from build123d import *

# Parameters (mm, degrees)
SKETCH1_R               = 15.875
SKETCH1_R_2             = 3.25
BOSS_EXTRUDE1_DEPTH     = 12.7
BOSS_EXTRUDE2_START     = -12.7
SKETCH1_3_W             = 38.1
SKETCH1_3_H             = 31.75
SKETCH1_3_R             = 3.25
BOSS_EXTRUDE2_DEPTH     = 12.7
CUT_EXTRUDE1_REACH      = 41.144
CUT_EXTRUDE1_END_RADIUS = 3.25
BOSS_EXTRUDE3_DEPTH     = 31.75
FILLET1_R               = 15.875
SKETCH8_R               = 6.35
CUT_EXTRUDE3_DEPTH      = 76.282979766
SKETCH8_3_R             = 9.5
SKETCH8_3_R_2           = 6.35
CUT_EXTRUDE4_DEPTH      = 6
SKETCH9_R               = 6.35
SKETCH9_R_2             = 5.5
BOSS_EXTRUDE4_DEPTH     = 13.05
SKETCH10_R              = 1.95
CUT_EXTRUDE5_DEPTH      = 10.16
CUT_EXTRUDE6_REACH      = 102.653
CUT_EXTRUDE6_END_RADIUS = 5.5


with BuildPart() as part:
    # Sketch1 → Boss-Extrude1 (new body)
    with BuildSketch(Plane.XY):
        Circle(SKETCH1_R)
        Circle(SKETCH1_R_2, mode=Mode.SUBTRACT)
    extrude(amount=BOSS_EXTRUDE1_DEPTH)

    # Sketch1<3> → Boss-Extrude2 (add)
    with BuildSketch(Plane.XY.offset(BOSS_EXTRUDE2_START)):
        Rectangle(SKETCH1_3_W, SKETCH1_3_H)
        Circle(SKETCH1_3_R, mode=Mode.SUBTRACT)
    extrude(amount=BOSS_EXTRUDE2_DEPTH)

    # Cut-Extrude1: up to this cylinder (the profile starts outside it)
    cut_extrude1_end = Plane(origin=(0, 0, 6.35), z_dir=(0, 0, -1)) * Cylinder(CUT_EXTRUDE1_END_RADIUS, 89.788, mode=Mode.PRIVATE)
    # Sketch4 → Cut-Extrude1 (cut, up to the surface)
    with BuildSketch(Plane(origin=(0, 15.875, 0), x_dir=(1, 0, 0), z_dir=(0, 1, 0)), mode=Mode.PRIVATE) as cut_extrude1_sk1:
        with BuildLine():
            ThreePointArc((1.95, -6.35), (1.378858223, -4.971141777), (0, -4.4))
            Line((0, -4.4), (0, -8.3))
            ThreePointArc((0, -8.3), (1.378858223, -7.728858223), (1.95, -6.35))
        make_face()
    cut_extrude1_tool1 = extrude(cut_extrude1_sk1.sketch, amount=-CUT_EXTRUDE1_REACH, mode=Mode.PRIVATE) - cut_extrude1_end
    add(cut_extrude1_tool1.solids().sort_by_distance((0.827606, 15.875, 6.35))[0], mode=Mode.SUBTRACT)
    # Sketch4 → Cut-Extrude1 (cut, up to the surface)
    with BuildSketch(Plane(origin=(0, 15.875, 0), x_dir=(1, 0, 0), z_dir=(0, 1, 0)), mode=Mode.PRIVATE) as cut_extrude1_sk2:
        with BuildLine():
            Line((0, -8.3), (0, -4.4))
            ThreePointArc((0, -4.4), (-1.95, -6.35), (0, -8.3))
        make_face()
    cut_extrude1_tool2 = extrude(cut_extrude1_sk2.sketch, amount=-CUT_EXTRUDE1_REACH, mode=Mode.PRIVATE) - cut_extrude1_end
    add(cut_extrude1_tool2.solids().sort_by_distance((-0.827606, 15.875, 6.35))[0], mode=Mode.SUBTRACT)
    # Sketch4 → Cut-Extrude1 (cut, up to the surface)
    with BuildSketch(Plane(origin=(0, 15.875, 0), x_dir=(1, 0, 0), z_dir=(0, 1, 0)), mode=Mode.PRIVATE) as cut_extrude1_sk3:
        with BuildLine():
            ThreePointArc((1.95, -6.35), (1.378858223, -4.971141777), (0, -4.4))
            Line((0, -4.4), (0, -8.3))
            ThreePointArc((0, -8.3), (1.378858223, -7.728858223), (1.95, -6.35))
        make_face()
    cut_extrude1_tool3 = extrude(cut_extrude1_sk3.sketch, amount=-CUT_EXTRUDE1_REACH, mode=Mode.PRIVATE) - cut_extrude1_end
    add(cut_extrude1_tool3.solids().sort_by_distance((0.827606, 15.875, 6.35))[0], mode=Mode.SUBTRACT)
    # Sketch4 → Cut-Extrude1 (cut, up to the surface)
    with BuildSketch(Plane(origin=(0, 15.875, 0), x_dir=(1, 0, 0), z_dir=(0, 1, 0)), mode=Mode.PRIVATE) as cut_extrude1_sk4:
        with BuildLine():
            Line((0, -8.3), (0, -4.4))
            ThreePointArc((0, -4.4), (-1.95, -6.35), (0, -8.3))
        make_face()
    cut_extrude1_tool4 = extrude(cut_extrude1_sk4.sketch, amount=-CUT_EXTRUDE1_REACH, mode=Mode.PRIVATE) - cut_extrude1_end
    add(cut_extrude1_tool4.solids().sort_by_distance((-0.827606, 15.875, 6.35))[0], mode=Mode.SUBTRACT)

    # Sketch7 → Boss-Extrude3 (add)
    with BuildSketch(Plane(origin=(0, 15.875, 0), x_dir=(1, 0, 0), z_dir=(0, 1, 0))):
        with BuildLine():
            ThreePointArc((-19.05, 12.7), (-23.740191201, 19.121901724), (-25.4, 26.899031657))
            Line((-25.4, 26.899031657), (-25.4, 58.649031657))
            Line((-25.4, 58.649031657), (-44.45, 58.649031657))
            Line((-44.45, 58.649031657), (-44.45, 31.75))
            ThreePointArc((-44.45, 31.75), (-37.318649317, 11.420080546), (-19.05, 0))
            Line((-19.05, 0), (-19.05, 12.7))
        make_face()
    extrude(amount=-BOSS_EXTRUDE3_DEPTH)

    # Fillet1
    fillet1_edges = [part.edges().sort_by_distance(p)[0] for p in [
        (-34.925, -15.875, -58.649031657),
        (-34.925, 15.875, -58.649031657),
    ]]
    fillet(fillet1_edges, radius=FILLET1_R - 0.0001)  # a hair under: the kernel refuses the full size

    # Sketch8 → Cut-Extrude3 (cut, through all)
    with BuildSketch(Plane(origin=(-25.4, 0, 0), x_dir=(0, 0, -1), z_dir=(1, 0, 0))):
        with Locations((42.774031657, 0)):
            Circle(SKETCH8_R)
    extrude(amount=-CUT_EXTRUDE3_DEPTH, mode=Mode.SUBTRACT)

    # Sketch8<3> → Cut-Extrude4 (cut)
    with BuildSketch(Plane(origin=(-25.4, 0, 0), x_dir=(0, 0, -1), z_dir=(1, 0, 0))):
        with Locations((42.774031657, 0)):
            Circle(SKETCH8_3_R)
        with Locations((42.774031657, 0)):
            Circle(SKETCH8_3_R_2, mode=Mode.SUBTRACT)
    extrude(amount=-CUT_EXTRUDE4_DEPTH, mode=Mode.SUBTRACT)

    # Mirror1: part across plane


with BuildPart() as part_1:
    add(part.part)
    add(part.part.mirror(Plane(origin=(0, 0, 0), x_dir=(0, 0, 1), z_dir=(1, 0, 0))))

    # Sketch9 → Boss-Extrude4 (add)
    with BuildSketch(Plane(origin=(44.45, 0, 0), x_dir=(0, 0, -1), z_dir=(1, 0, 0))):
        with Locations((42.774031657, 0)):
            Circle(SKETCH9_R)
        with Locations((42.774031657, 0)):
            Circle(SKETCH9_R_2, mode=Mode.SUBTRACT)
    extrude(amount=-BOSS_EXTRUDE4_DEPTH)

    # Sketch10 → Cut-Extrude5 (cut)
    with BuildSketch(Plane.ZY.offset(44.45)):
        with Locations((-42.774031657, 12.7)):
            Circle(SKETCH10_R)
        with Locations((-42.774031657, -12.7)):
            Circle(SKETCH10_R)
    extrude(amount=-CUT_EXTRUDE5_DEPTH, mode=Mode.SUBTRACT)

    # Cut-Extrude6: up to this cylinder (the profile starts outside it)
    cut_extrude6_end = Plane(origin=(35.381138, 0, -42.774031657), z_dir=(1, 0, 0)) * Cylinder(CUT_EXTRUDE6_END_RADIUS, 217.306, mode=Mode.PRIVATE)
    # Sketch11 → Cut-Extrude6 (cut, up to the surface)
    with BuildSketch(Plane.XY.offset(-76.2), mode=Mode.PRIVATE) as cut_extrude6_sk1:
        with BuildLine():
            ThreePointArc((33.431138122, 0), (35.381138122, -1.95), (37.331138122, 0))
            Line((37.331138122, 0), (33.431138122, 0))
        make_face()
    cut_extrude6_tool1 = extrude(cut_extrude6_sk1.sketch, amount=CUT_EXTRUDE6_REACH, mode=Mode.PRIVATE) - cut_extrude6_end
    add(cut_extrude6_tool1.solids().sort_by_distance((35.381138, -0.827606, -76.2))[0], mode=Mode.SUBTRACT)
    # Sketch11 → Cut-Extrude6 (cut, up to the surface)
    with BuildSketch(Plane.XY.offset(-76.2), mode=Mode.PRIVATE) as cut_extrude6_sk2:
        with BuildLine():
            Line((33.431138122, 0), (37.331138122, 0))
            ThreePointArc((37.331138122, 0), (35.381138122, 1.95), (33.431138122, 0))
        make_face()
    cut_extrude6_tool2 = extrude(cut_extrude6_sk2.sketch, amount=CUT_EXTRUDE6_REACH, mode=Mode.PRIVATE) - cut_extrude6_end
    add(cut_extrude6_tool2.solids().sort_by_distance((35.381138, 0.827606, -76.2))[0], mode=Mode.SUBTRACT)
    # Sketch11 → Cut-Extrude6 (cut, up to the surface)
    with BuildSketch(Plane.XY.offset(-76.2), mode=Mode.PRIVATE) as cut_extrude6_sk3:
        with BuildLine():
            ThreePointArc((33.431138122, 0), (35.381138122, -1.95), (37.331138122, 0))
            Line((37.331138122, 0), (33.431138122, 0))
        make_face()
    cut_extrude6_tool3 = extrude(cut_extrude6_sk3.sketch, amount=CUT_EXTRUDE6_REACH, mode=Mode.PRIVATE) - cut_extrude6_end
    add(cut_extrude6_tool3.solids().sort_by_distance((35.381138, -0.827606, -76.2))[0], mode=Mode.SUBTRACT)
    # Sketch11 → Cut-Extrude6 (cut, up to the surface)
    with BuildSketch(Plane.XY.offset(-76.2), mode=Mode.PRIVATE) as cut_extrude6_sk4:
        with BuildLine():
            Line((33.431138122, 0), (37.331138122, 0))
            ThreePointArc((37.331138122, 0), (35.381138122, 1.95), (33.431138122, 0))
        make_face()
    cut_extrude6_tool4 = extrude(cut_extrude6_sk4.sketch, amount=CUT_EXTRUDE6_REACH, mode=Mode.PRIVATE) - cut_extrude6_end
    add(cut_extrude6_tool4.solids().sort_by_distance((35.381138, 0.827606, -76.2))[0], mode=Mode.SUBTRACT)


solid = part_1.part
Design review of the part built by this model. Coordinates are the model's own, in mm. A direction names the side the tool comes from. Coordinates: 2 decimals unless noted, no trailing zeros. Write each loop counter-clockwise with the first axis right and the second up, starting at its lowest first coordinate (ties: lowest second). Pieces come first, ordered by that corner, then holes. Notation, with made-up numbers: (14.25, -13) -> (71.25, -13) arc R8 ccw to (71.25, -7) -> close; hole circle Ø5 at (-35.5, 56.5). An arc over 180 degrees is marked (long way). Write each question's results on one line, items separated by ' | '. Start each with the question number.
(1) For line 1 along X through (y, z) = (4.5, -32.5); line 2 along X through (y, z) = (1.5, -36); line 3 along Z through (x, y) = (-15.5, 5.5), list the stretches that pass through material, from the lowest coordinate up. Write a range as from..to.
(2) The part is to be moulded in two halves that separate along Y. For faces 1 (the face through (0, 4, 12.7)), 2 (the face through (38.02, -3.35, -38.41)), 3 (the face through (-35.058, -11.348, -53.875)), 4 (the face through (-34.29, 13, -43)), say which applies: pulls with the +Y half, pulls with the -Y half, needs draft (parallel to the pull), parting line crosses it, or undercut.
(3) Take a section at D-D on x = -39. Give the number of separate pieces and of enclosed holes in the cut face, and give its area (3 significant figures).
(4) Tool access review of faces 5 (the face through (-25.4, -7, -35)), 6 (the face through (16, -2, 0)), 7 (the face through (-37.83, 1.91, -48.83)): name each direction out of +Z, -Z, +X, -X, +Y, -Y from which nothing blocks a thin tool from reaching the whole face with its end or side.
(5) Take a section at A-A on z = -28. Write out the cut boundary in (x, y) (3 decimals), and give its area (3 significant figures).
(6) Clearance check with flat-ended pins moving along their axes: P1, Ø6, axis at x = -24.5, y = -8, coming from the -Z side; P2, Ø3.5, axis at x = 35.38, y = 0, coming from the -Z side; P3, Ø1.5, axis at y = -2, z = -23.5, coming from the -X side. State where each tip first meets the part, or that it passes through.
Results found:
1) line 1: x = -44.45..-25.4, 25.4..44.45 | line 2: x = -44.45..-31.4, 31.4..44.45 | line 3: z = -12.7..0
2) face 1: needs draft | face 2: undercut | face 3: pulls with the -Y half | face 4: undercut
3) separate pieces: 1 | enclosed holes: 3 | area: 1,170 mm2
4) face 5: -Z, +Y, -Y | face 6: +Z, +X | face 7: -X
5) outline: (-44.233, -15.875) -> (-25.4, -15.875) -> (-25.4, 15.875) -> (-44.233, 15.875) -> close; (25.4, -15.875) -> (44.233, -15.875) -> (44.233, 15.875) -> (25.4, 15.875) -> close | area: 1,200 mm2
6) P1: stops at z = -57.79 | P2: stops at z = -37.56 | P3: stops at x = -43.57
